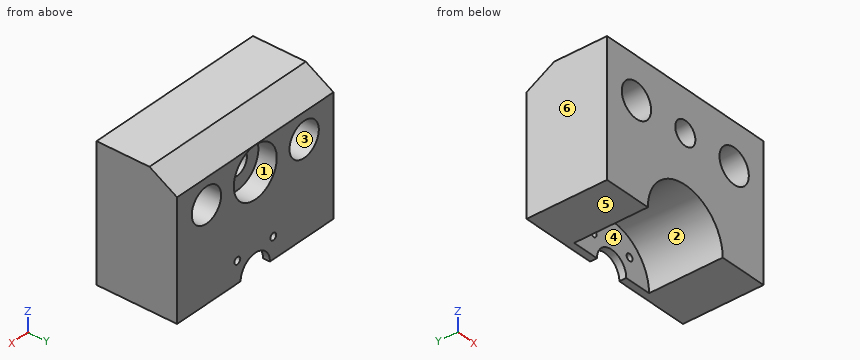
```python
from build123d import *

# Parameters (mm, degrees)
BOSS_EXTRUDE1_DEPTH = 35
SKETCH2_R           = 7.5
SKETCH2_R_2         = 5.15
CUT_EXTRUDE1_DEPTH  = 36
BOSS_EXTRUDE2_DEPTH = 3
SKETCH6_R           = 1.5
CUT_EXTRUDE3_DEPTH  = 4
CHAMFER1_SIZE       = 12
CHAMFER1_SIZE2      = 6.92820323
SKETCH7_R           = 11
CUT_EXTRUDE4_DEPTH  = 8


with BuildPart() as part:
    # Sketch1 → Boss-Extrude1 (new body)
    with BuildSketch(Plane(origin=(0, 0, 0), x_dir=(1, 0, 0), z_dir=(0, 1, 0))):
        with BuildLine():
            Line((19.15, 0), (40, 0))
            Line((40, 0), (40, -58))
            Line((40, -58), (-40, -58))
            Line((-40, -58), (-40, 0))
            Line((-40, 0), (-19.15, 0))
            ThreePointArc((-19.15, 0), (0, -19.15), (19.15, 0))
        make_face()
    extrude(amount=BOSS_EXTRUDE1_DEPTH)

    # Sketch2 → Cut-Extrude1 (cut, through all)
    with BuildSketch(Plane(origin=(0, 35, 0), x_dir=(1, 0, 0), z_dir=(0, 1, 0))):
        with Locations((-25, -40)):
            Circle(SKETCH2_R)
        with Locations((25, -40)):
            Circle(SKETCH2_R)
        with Locations((0, -40)):
            Circle(SKETCH2_R_2)
    extrude(amount=-CUT_EXTRUDE1_DEPTH, mode=Mode.SUBTRACT)

    # Sketch5 → Boss-Extrude2 (add)
    with BuildSketch(Plane(origin=(0, 35, 0), x_dir=(1, 0, 0), z_dir=(0, 1, 0))):
        with BuildLine():
            Line((-19.15, 0), (-7.5, 0))
            ThreePointArc((-7.5, 0), (0, -7.5), (7.5, 0))
            Line((7.5, 0), (19.15, 0))
            ThreePointArc((19.15, 0), (0, -19.15), (-19.15, 0))
        make_face()
    extrude(amount=-BOSS_EXTRUDE2_DEPTH)

    # Sketch6 → Cut-Extrude3 (cut, through all)
    with BuildSketch(Plane.XZ.offset(-32)):
        with Locations((9.192388155, 9.192388155)):
            Circle(SKETCH6_R)
        with Locations((-9.192388155, 9.192388155)):
            Circle(SKETCH6_R)
    extrude(amount=-CUT_EXTRUDE3_DEPTH, mode=Mode.SUBTRACT)

    # Chamfer1
    chamfer1_edges = [part.edges().sort_by_distance(p)[0] for p in [
        (0, 35, 58),
    ]]
    chamfer1_side = [part.faces().sort_by_distance(p)[0] for p in [
        (0, 17.5, 58),
    ]]
    chamfer(chamfer1_edges, length=CHAMFER1_SIZE, length2=CHAMFER1_SIZE2, reference=chamfer1_side[0])

    # Sketch7 → Cut-Extrude4 (cut)
    with BuildSketch(Plane(origin=(0, 35, 0), x_dir=(1, 0, 0), z_dir=(0, 1, 0))):
        with Locations((0, -40)):
            Circle(SKETCH7_R)
    extrude(amount=-CUT_EXTRUDE4_DEPTH, mode=Mode.SUBTRACT)


solid = part.part
```
CAD build for the part. Positions are in the model's coordinates, mm. Face numbers are marked on the shaded views. A direction names the side the tool comes from. Coordinates: 2 decimals unless noted, no trailing zeros. Write each loop counter-clockwise with the first axis right and the second up, starting at its lowest first coordinate (ties: lowest second). Pieces come first, ordered by that corner, then holes.
(1) 3-axis set-ups, long thin cutter, end or side, ignore diameter. For the marked faces 1, 2 and 3: which of +Z, -Z, +X, -X, +Y, -Y reach the whole face in a straight line?
(2) Cut at A-A, the plane x = 0. List the corners of the cut face in (y, z).
(3) Two-plate mould, pull along X, no slides. Class the marked faces 4, 5 and 6: +X half, -X half, draft (parallel to the pull), parting line (faces both ways), or undercut.
(4) Drill centre lines: probe 1 along X at (y, z) = (12, 43); probe 2 along X at (y, z) = (30, 36); probe 3 along Y at (x, z) = (-1, 48). Where is each one in solid material? Low to high.
(5) Cut at D-D, the plane x = -25. List the corners of the cut face in (y, z), and give its area (3 significant figures).
(6) Flat gauge pins, fed straight in: pin 1 (6 mm diameter, centred on x = 0, z = 40, fed in from -Y); pin 2 (5 mm diameter, centred on x = -9.19, z = 9.19, fed in from -Y). Where does each tip first touch, or does it go through?
(7) Cut at B-B, the plane z = 40. List the corners of the cut face in (x, y), and give its area (3 significant figures).
(8) Cut at C-C, the plane y = 9.5. List the corners of the cut face in (x, z), and give its area (3 significant figures).
Geometry says:
1. face 1: +Y
1. face 2: -Z, -Y
1. face 3: +Y, -Y
2. outline: (0, 19.15) - (32, 19.15) - (32, 7.5) - (35, 7.5) - (35, 29) - (27, 29) - (27, 34.85) - (0, 34.85) - close; (0, 45.15) - (27, 45.15) - (27, 51) - (35, 51) - (35, 51.07) - (23, 58) - (0, 58) - close
3. face 4: undercut
3. face 5: draft
3. face 6: -X half
4. probe 1: x = -40 to -31.87, -18.13 to -4.19, 4.19 to 18.13, 31.87 to 40
4. probe 2: x = -40 to -31.34, -18.66 to -10.25, 10.25 to 18.66, 31.34 to 40
4. probe 3: y = 0 to 27
5. outline: (0, 0) - (35, 0) - (35, 32.5) - (0, 32.5) - close; (0, 47.5) - (35, 47.5) - (35, 51.07) - (23, 58) - (0, 58) - close
5. area: 1,460 mm2
6. pin 1: passes through
6. pin 2: stops at y = 32
7. outline: (-40, 0) - (-32.5, 0) - (-32.5, 35) - (-40, 35) - close; (-17.5, 0) - (-5.15, 0) - (-5.15, 27) - (-11, 27) - (-11, 35) - (-17.5, 35) - close; (5.15, 0) - (17.5, 0) - (17.5, 35) - (11, 35) - (11, 27) - (5.15, 27) - close; (32.5, 0) - (40, 0) - (40, 35) - (32.5, 35) - close
7. area: 1,300 mm2
8. outline: (-40, 0) - (-19.15, 0) arc R19.15 cw to (19.15, 0) - (40, 0) - (40, 58) - (-40, 58) - close; hole circle Ø15 at (-25, 40); hole circle Ø10.3 at (0, 40); hole circle Ø15 at (25, 40)
8. area: 3,630 mm2
